Could you check a few things on this model? Use its own coordinates, in mm. A direction names the side the tool comes from. Give positions to 0.01 mm unless a question says otherwise; leave off trailing zeros. Write each loop counter-clockwise with the first axis right and the second up, starting at its lowest first coordinate (ties: lowest second). Pieces come first, ordered by that corner, then holes. Notation, with made-up numbers: (7, 5) - (59, 5) arc R26 ccw to (59, 31) - close; hole circle Ø8 at (14, 61.5). An arc over 180 degrees is marked (long way). Write item = value, one per line.
from build123d import *

# Parameters (mm, degrees)
F0_W     = 100
F0_H     = 100
F0_R     = 2.5
F1_DEPTH = 10
F2_R     = 2.5
F3_DEPTH = 5


with BuildPart() as f1:
    # F0 (on Front) → F1 (new body)
    with BuildSketch(Plane.XZ):
        with Locations((50, 50)):
            Rectangle(F0_W, F0_H)
        with Locations((12, 81.869952)):
            Circle(F0_R, mode=Mode.SUBTRACT)
        with Locations((29, 81.869952)):
            Circle(F0_R, mode=Mode.SUBTRACT)
        with Locations((48, 81.869952)):
            Circle(F0_R, mode=Mode.SUBTRACT)
        with Locations((69, 81.869952)):
            Circle(F0_R, mode=Mode.SUBTRACT)
        with Locations((12, 81.869952)):
            Circle(F0_R)
        with Locations((29, 81.869952)):
            Circle(F0_R)
        with Locations((48, 81.869952)):
            Circle(F0_R)
        with Locations((69, 81.869952)):
            Circle(F0_R)
    extrude(amount=F1_DEPTH)

    # F2 (on face) → F3 (join)
    with BuildSketch(Plane.XZ.offset(10)):
        with Locations((18, 82.490392)):
            Circle(F2_R)
        with Locations((35, 82.490392)):
            Circle(F2_R)
        with Locations((54, 82.490392)):
            Circle(F2_R)
        with Locations((75, 82.490392)):
            Circle(F2_R)
        with Locations((75, 59.490392)):
            Circle(F2_R)
        with Locations((75, 34.490392)):
            Circle(F2_R)
        with Locations((48, 34.490392)):
            Circle(F2_R)
    extrude(amount=F3_DEPTH)


solid = f1.part
1. I need wall thicknesses on line 1 (Y direction, x = 29, z = 44.5); line 2 (Z direction, x = 18, y = -10.25); line 3 (X direction, y = -13, z = 36.5). Which ranges of each line are inside material? Lowest first, please.
Filled sheet:
line_1 = -10 to 0
line_2 = 79.99 to 84.99
line_3 = 46.51 to 49.49, 73.51 to 76.49
2. If we section it at D-D, the plane z = 94: Please give me the cut outline in (x, y).
Filled sheet:
outline = (0, -10) - (100, -10) - (100, 0) - (0, 0) - close
3. If we section it at C-C, the plane x = 75: Please give me the cut outline in (y, z), and give its area (4 significant figures).
Filled sheet:
outline = (-15, 31.99) - (-10, 31.99) - (-10, 0) - (0, 0) - (0, 100) - (-10, 100) - (-10, 84.99) - (-15, 84.99) - (-15, 79.99) - (-10, 79.99) - (-10, 61.99) - (-15, 61.99) - (-15, 56.99) - (-10, 56.99) - (-10, 36.99) - (-15, 36.99) - close
area = 1,075 mm2
4. If we section it at B-B, the plane y = -12.75: Please give me the cut outline in (x, z).
Filled sheet:
outline = circle Ø5 at (18, 82.49); circle Ø5 at (35, 82.49); circle Ø5 at (48, 34.49); circle Ø5 at (54, 82.49); circle Ø5 at (75, 34.49); circle Ø5 at (75, 59.49); circle Ø5 at (75, 82.49)
5. If we section it at A-A, the plane x = 18: Please give me the cut outline in (y, z).
Filled sheet:
outline = (-15, 79.99) - (-10, 79.99) - (-10, 0) - (0, 0) - (0, 100) - (-10, 100) - (-10, 84.99) - (-15, 84.99) - close
6. Thinking about a two-plate mould opening in X: for faces 1 (the face through (35, -15, 83)), 2 (the face through (0, -5, 49)), 3 (the face through (74.46, -12.46, 80.05)), which applies, pulls with the +X half, pulls with the -X half, needs draft (parallel to the pull), parting line crosses it, or undercut?
Filled sheet:
face_1 = needs draft
face_2 = pulls with the -X half
face_3 = undercut
7. For pin 1 (3 mm diameter, centred on x = 75, y = -10.5, fed in from -Z), with a flat end and sliding along its axis, tell me the tip position at first contact or that it passes through.
Filled sheet:
pin_1 = 0
8. Which directions (+Z, -Z, +X, -X, +Y, -Y) give clear straight access to the entire face, cutting with the end or side of a thin tool? Please do faces 4 (the face through (73.016, -12.465, 32.969)), 5 (the face through (100, -5, 49)).
Filled sheet:
face_4 = -Y
face_5 = +Z, -Z, +X, +Y, -Y
